```python
from build123d import *

# Parameters (mm, degrees)
SKETCH_1_R           = 1.5
EXTRUDE_1_DEPTH      = 3
EXTRUDE_2_DEPTH      = 3
EXTRUDE_2_DEPTH_BACK = 3
SKETCH_2_R           = 1.5


with BuildPart() as part:
    # Sketch 1 → Extrude 1 (new body)
    with BuildSketch(Plane(origin=(0, 0, 0), x_dir=(1, 0, 0), z_dir=(0, 1, 0))):
        with BuildLine():
            Line((-96.621430383, 38.303370954), (-70.818390196, 45.39148714))
            ThreePointArc((-70.818390196, 45.39148714), (-73.937652642, 15.166954083), (-98.553234864, -2.646672965))
            Line((-98.553234864, -2.646672965), (-105.316266275, 23.243473425))
            ThreePointArc((-105.316266275, 23.243473425), (-97.009577473, 28.487536095), (-96.621430383, 38.303370954))
        make_face()
        with Locations(Location((-86.118640655, 5.183838281, 0), (0, 0, 270))):
            Circle(SKETCH_1_R, mode=Mode.SUBTRACT)
        with Locations(Location((-71.373114162, 30.69577881, 0), (0, 0, 270))):
            Circle(SKETCH_1_R, mode=Mode.SUBTRACT)
    extrude(amount=EXTRUDE_1_DEPTH)

    # Sketch 2 → Extrude 2 (add, two sides: drawn at the far end of the back side and taken through both)
    with BuildSketch(Plane(origin=(0, 3, 0), x_dir=(1, 0, 0), z_dir=(0, 1, 0)).offset(-EXTRUDE_2_DEPTH_BACK)):
        with Locations(Location((-71.373114162, 30.69577881, 0), (0, 0, 270))):
            Circle(SKETCH_2_R)
        with Locations(Location((-86.118640655, 5.183838281, 0), (0, 0, 270))):
            Circle(SKETCH_2_R)
    extrude(amount=EXTRUDE_2_DEPTH + EXTRUDE_2_DEPTH_BACK)


solid = part.part
```
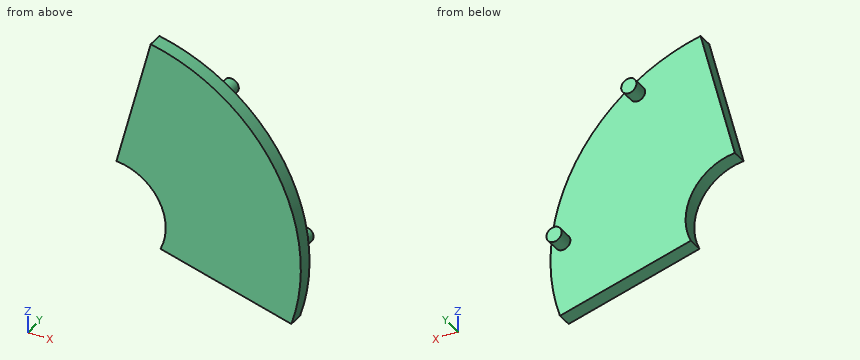
CAD build for the part. Positions are in the model's coordinates, mm. Round coordinates to 2 decimals unless told otherwise and drop trailing zeros. Order: outer loops, then holes, each group sorted by start corner. A loop starts at its lowest first (then second) coordinate and runs counter-clockwise, first axis right, second up. Notation, with made-up numbers: (30.25, 30) -> (50.25, 30) arc R30 cw to (50.25, 56) -> close; hole circle Ø5 at (56.25, 50). An arc over 180 degrees is marked (long way). Write item = value, one per line.
(1) Cut at A-A (x = -85.5). Write the cut outline in (y, z), plus the area to 3 significant figures.
Answers follow:
outline = (0, -41.36) -> (3, -41.36) -> (3, -6.55) -> (6, -6.55) -> (6, -3.82) -> (3, -3.82) -> (3, -2.83) -> (0, -2.83) -> close
area = 124 mm²
(2) Flat gauge pins, fed straight in: P1, Ø1, axis at x = -97.5, z = -21.5, coming from the +Y side; P2, Ø1, axis at y = 1.5, z = -26, coming from the +X side. Where does each tip first touch, or does it go through?
Answers follow:
P1 = 3
P2 = -69.67
(3) Cut at C-C (y = 0.7). Write the cut outline in (x, z), plus the area to 3 significant figures.
Answers follow:
outline = (-105.32, -23.24) arc R10.55 cw to (-96.62, -38.3) -> (-70.82, -45.39) arc R37.2 ccw to (-98.55, 2.65) -> close
area = 1,110 mm²
(4) Drill centre lines: L1, parallel to Y at x = -89, z = -24; L2, parallel to X at y = 0.9, z = -14.5; L3, parallel to X at y = 1.7, z = -12.5. Where is each one in solid material? Low to high.
Answers follow:
L1 = 0 to 3
L2 = -103.03 to -74.33
L3 = -102.51 to -75.63
(5) Cut at D-D (z = -16.5). Write the cut outline in (x, y).
Answers follow:
outline = (-103.55, 0) -> (-73.2, 0) -> (-73.2, 3) -> (-103.55, 3) -> close
(6) Cut at B-B (y = 3.8). Write the cut outline in (x, z), plus the area to 3 significant figures.
Answers follow:
outline = circle Ø3 at (-86.12, -5.18); circle Ø3 at (-71.37, -30.7)
area = 14.1 mm²
